from build123d import *

# Parameters (mm, degrees)
SKETCH_1_R               = 1.5
EXTRUDE_1_DEPTH          = 2
SKETCH_2_R               = 1.5
CUT_EXTRUDE_1_DEPTH      = 151.628682528
SKETCH_3_W               = 278
SKETCH_3_H               = 20
CUT_EXTRUDE_2_DEPTH      = 151.628682528
CUT_EXTRUDE_3_DEPTH      = 151.628682528
CUT_EXTRUDE_3_DEPTH_BACK = 151.628682528


with BuildPart() as part:
    # 草图1 → 凸台-拉伸1 (new body)
    with BuildSketch(Plane.XY):
        Polygon((-101, 30), (-101, 0), (101, 0), (101, 30), (139, 30), (139, 0), (81, -58), (-81, -58), (-139, 0), (-139, 30), align=None)
        with Locations((-135, 25)):
            Circle(SKETCH_1_R, mode=Mode.SUBTRACT)
        with Locations((-105, 25)):
            Circle(SKETCH_1_R, mode=Mode.SUBTRACT)
        with Locations((-105, 5)):
            Circle(SKETCH_1_R, mode=Mode.SUBTRACT)
        with Locations((-135, 5)):
            Circle(SKETCH_1_R, mode=Mode.SUBTRACT)
        with Locations(Location((135, 5, 0), (0, 0, 180))):
            Circle(SKETCH_1_R, mode=Mode.SUBTRACT)
        with Locations(Location((105, 5, 0), (0, 0, 180))):
            Circle(SKETCH_1_R, mode=Mode.SUBTRACT)
        with Locations(Location((105, 25, 0), (0, 0, 180))):
            Circle(SKETCH_1_R, mode=Mode.SUBTRACT)
        with Locations(Location((135, 25, 0), (0, 0, 180))):
            Circle(SKETCH_1_R, mode=Mode.SUBTRACT)
        with Locations((-70, -53)):
            Circle(SKETCH_1_R, mode=Mode.SUBTRACT)
        with Locations((-50, -53)):
            Circle(SKETCH_1_R, mode=Mode.SUBTRACT)
        with Locations(Location((50, -53, 0), (0, 0, 180))):
            Circle(SKETCH_1_R, mode=Mode.SUBTRACT)
        with Locations(Location((70, -53, 0), (0, 0, 180))):
            Circle(SKETCH_1_R, mode=Mode.SUBTRACT)
    extrude(amount=EXTRUDE_1_DEPTH)

    # 草图2 → 切除-拉伸1 (cut, through all)
    with BuildSketch(Plane.XY.offset(2)):
        with Locations((-105.142135624, -28.201010127)):
            Circle(SKETCH_2_R)
        with Locations((-91, -42.343145751)):
            Circle(SKETCH_2_R)
        with Locations(Location((91, -42.343145751, 0), (0, 0, 180))):
            Circle(SKETCH_2_R)
        with Locations(Location((105.142135624, -28.201010127, 0), (0, 0, 180))):
            Circle(SKETCH_2_R)
    extrude(amount=-CUT_EXTRUDE_1_DEPTH, mode=Mode.SUBTRACT)

    # 草图3 → 切除-拉伸2 (cut, through all)
    with BuildSketch(Plane.XY.offset(2)):
        with Locations((0, 20)):
            Rectangle(SKETCH_3_W, SKETCH_3_H)
    extrude(amount=-CUT_EXTRUDE_2_DEPTH, mode=Mode.SUBTRACT)

    # 草图4 → 切除-拉伸3 (cut, two sides: drawn at the far end of the back side and taken through both)
    with BuildSketch(Plane.XY.offset(2).offset(-CUT_EXTRUDE_3_DEPTH_BACK)):
        with BuildLine():
            Line((-105.226136393, -12.560660172), (-83.560660172, -34.226136393))
            ThreePointArc((-83.560660172, -34.226136393), (-81.925974851, -34.55129552), (-81, -33.165476221))
            Line((-81, -33.165476221), (-81, -11.5))
            ThreePointArc((-81, -11.5), (-81.439339828, -10.439339828), (-82.5, -10))
            Line((-82.5, -10), (-104.165476221, -10))
            ThreePointArc((-104.165476221, -10), (-105.55129552, -10.925974851), (-105.226136393, -12.560660172))
        make_face()
        with BuildLine():
            Line((-73, -19), (-73, -43.286796564))
            ThreePointArc((-73, -43.286796564), (-72.560660172, -44.347456736), (-71.5, -44.786796564))
            Line((-71.5, -44.786796564), (-39.117604581, -44.786796564))
            ThreePointArc((-39.117604581, -44.786796564), (-37.694579634, -43.761138213), (-38.217604581, -42.086796564))
            Line((-38.217604581, -42.086796564), (-70.6, -17.8))
            ThreePointArc((-70.6, -17.8), (-72.170820393, -17.658359214), (-73, -19))
        make_face()
        with BuildLine():
            Line((-63.166666667, -10), (-8, -10))
            ThreePointArc((-8, -10), (-6.644239805, -10.858194505), (-6.839820875, -12.450780941))
            Line((-6.839820875, -12.450780941), (-27.839820875, -38.075780941))
            ThreePointArc((-27.839820875, -38.075780941), (-28.819858864, -38.614143771), (-29.9, -38.325))
            Line((-29.9, -38.325), (-64.066666667, -12.7))
            ThreePointArc((-64.066666667, -12.7), (-64.589691614, -11.025658351), (-63.166666667, -10))
        make_face()
        with BuildLine():
            Line((29.9, -38.325), (64.066666667, -12.7))
            ThreePointArc((64.066666667, -12.7), (64.589691614, -11.025658351), (63.166666667, -10))
            Line((63.166666667, -10), (8, -10))
            ThreePointArc((8, -10), (6.644239805, -10.858194505), (6.839820875, -12.450780941))
            Line((6.839820875, -12.450780941), (27.839820875, -38.075780941))
            ThreePointArc((27.839820875, -38.075780941), (28.819858864, -38.614143771), (29.9, -38.325))
        make_face()
        with BuildLine():
            Line((38.217604581, -42.086796564), (70.6, -17.8))
            ThreePointArc((70.6, -17.8), (72.170820393, -17.658359214), (73, -19))
            Line((73, -19), (73, -43.286796564))
            ThreePointArc((73, -43.286796564), (72.560660172, -44.347456736), (71.5, -44.786796564))
            Line((71.5, -44.786796564), (39.117604581, -44.786796564))
            ThreePointArc((39.117604581, -44.786796564), (37.694579634, -43.761138213), (38.217604581, -42.086796564))
        make_face()
        with BuildLine():
            Line((82.5, -10), (104.165476221, -10))
            ThreePointArc((104.165476221, -10), (105.55129552, -10.925974851), (105.226136393, -12.560660172))
            Line((105.226136393, -12.560660172), (83.560660172, -34.226136393))
            ThreePointArc((83.560660172, -34.226136393), (81.925974851, -34.55129552), (81, -33.165476221))
            Line((81, -33.165476221), (81, -11.5))
            ThreePointArc((81, -11.5), (81.439339828, -10.439339828), (82.5, -10))
        make_face()
        with BuildLine():
            Line((-22.280808546, -42.336015623), (-1.160179125, -16.563819008))
            ThreePointArc((-1.160179125, -16.563819008), (0, -16.014599949), (1.160179125, -16.563819008))
            Line((1.160179125, -16.563819008), (22.280808546, -42.336015623))
            ThreePointArc((22.280808546, -42.336015623), (22.476389616, -43.92860206), (21.120629421, -44.786796564))
            Line((21.120629421, -44.786796564), (-21.120629421, -44.786796564))
            ThreePointArc((-21.120629421, -44.786796564), (-22.476389616, -43.92860206), (-22.280808546, -42.336015623))
        make_face()
    extrude(amount=CUT_EXTRUDE_3_DEPTH + CUT_EXTRUDE_3_DEPTH_BACK, mode=Mode.SUBTRACT)


solid = part.part
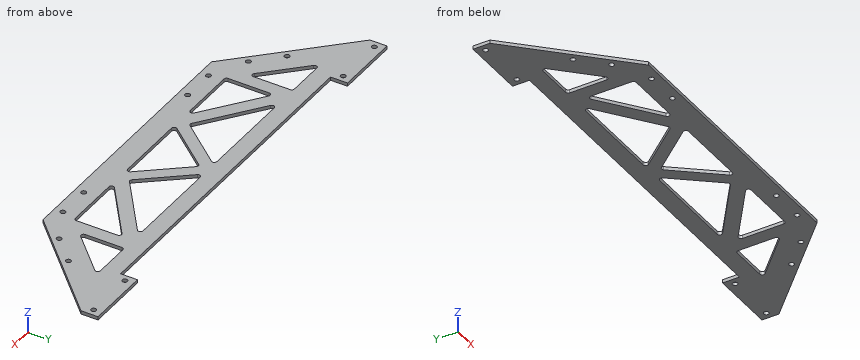
Verification items for the finished model (mm, model axes). Coordinates: 2 decimals unless noted, no trailing zeros. Write each loop counter-clockwise with the first axis right and the second up, starting at its lowest first coordinate (ties: lowest second). Pieces come first, ordered by that corner, then holes. Notation, with made-up numbers: M 83,15.5 L 98,15.5 A30 ccw 98,42.5 Z; hole C 65,-19 d8. An arc over 180 degrees is marked long. Use a Markdown table: item, result.
Q1. Thickness scan on line 1 (Y direction, x = 8.5, z = 1.7); line 2 (Y direction, x = -50, z = 1.35); line 3 (X direction, y = -41, z = 0.1). Record the ranges inside material, lowest first.
Reply:
| item | result |
|---|---|
| line 1 | y = -58 to -44.79, -25.52 to -14.48, -10 to 0 |
| line 2 | y = -58 to -54.5, -51.5 to -44.79, -33.25 to -23.25, -10 to 0 |
| line 3 | x = -98 to -91.67, -90.33 to -73, -39.67 to -21.19, 21.19 to 39.67, 73 to 90.33, 91.67 to 98 |
Q2. Go/stop test with flat-tipped pins: P1, Ø3.5, axis at x = -135, y = 5, coming from the +Z side; P2, Ø0.6, axis at x = -1.5, z = 1, coming from the +Y side; P3, Ø1, axis at y = -36.5, z = 1.5, coming from the +X side; P4, Ø1, axis at x = -90, z = 0.5, coming from the -Y side. Record where each tip stops, or that it passes through.
Reply:
| item | result |
|---|---|
| P1 | stops at z = 2 |
| P2 | stops at y = 0 |
| P3 | stops at x = 103 |
| P4 | stops at y = -49.5 |
Q3. Sectioned sample at B-B, the plane z = 0.5. Count the separate pieces of the cut face and the enclosed holes in it, plus the area to 3 significant figures.
Reply:
| item | result |
|---|---|
| separate pieces | 1 |
| enclosed holes | 19 |
| area | 9,100 mm² |
Q4. Sectioned sample at A-A, the plane x = 75.5. Record the boundary of the cut face in (y, z).
Reply:
| item | result |
|---|---|
| outline | M -58,0 L 0,0 L 0,2 L -58,2 Z |
